Verification items for the finished model (mm, model axes). Round coordinates to 2 decimals unless told otherwise and drop trailing zeros. Write each loop counter-clockwise with the first axis right and the second up, starting at its lowest first coordinate (ties: lowest second). Pieces come first, ordered by that corner, then holes. Notation, with made-up numbers: (81.25, 51.25) -> (86.25, 51.25) arc R26 cw to (86.25, 77.25) -> close; hole circle Ø3 at (47.25, 50). An arc over 180 degrees is marked (long way). Answer as a JSON object with one key per item and string values. Group by question number.
(1) Sectioned sample at A-A on y = -5. Record the cut outline in (x, z) (3 decimals), and give its area (3 significant figures).
(2) Scan lines: L1, parallel to X at y = 35, z = -1 (3 decimals); L2, parallel to Y at x = 84.5, z = -0.8; L3, parallel to X at y = 34, z = -0.4. Record each from-to range of solid material in increasing order. Write a range as from..to.
(3) Sectioned sample at D-D on z = -1.35. Count the separate pieces of the cut face and the enclosed holes in it, and give its area (3 significant figures).
(4) Gauge pin test, flat ends, axial feed: pin 1 Ø5 at (x, y) = (-114.625, 55.25) entering from +Z; pin 2 Ø24 at (x, y) = (90.125, 74) entering from +Z. Record the tip position at first contact, or that the pin passes through.
(5) Sectioned sample at B-B on x = 12.5. Record the cut outline in (y, z) (3 decimals).
(6) Sectioned sample at C-C on y = 65. Record the cut outline in (x, z) (3 decimals).
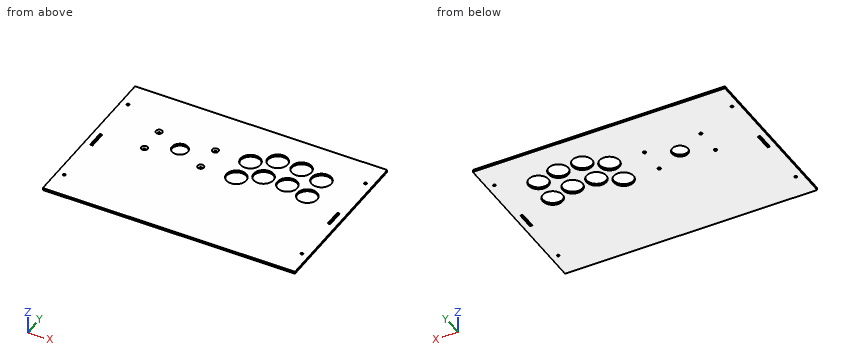
Autodesk Inventor part; units mm, degrees
ref_plane "YZ Plane" through (0, 0, 0) normal (1, 0, 0) x (0, 1, 0)
ref_plane "XZ Plane" through (0, 0, 0) normal (0, 1, 0) x (-1, 0, 0)
ref_plane "XY Plane" through (0, 0, 0) normal (0, 0, 1) x (1, 0, 0)
sketch "Panel" plane through (0, 0, 0) normal (0, 0, 1) x (1, 0, 0)
  line L0 (-190.5, 127) -> (190.5, 127)
  line L1 (190.5, 127) -> (190.5, -127)
  line L2 (190.5, -127) -> (-190.5, -127)
  line L3 (-190.5, -127) -> (-190.5, 127)
  point P0 (0, 0)
  point P1 (-190.5, 0)
  point P2 (0, 127)
  dimension "d0" = 254
  dimension "d3" = 381
sketch "JoystickMount" plane through (0, 0, 0) normal (0, 0, 1) x (1, 0, 0)
  line L0 (-114.625, 55.25) -> (-114.625, 14.75) construction
  line L1 (-114.625, 14.75) -> (-29.625, 14.75) construction
  point P0 (0, 0)
  point P1 (-72.125, 35)
  point P2 (-29.625, 55.25)
  point P3 (-114.625, 35)
  point P4 (-72.125, 14.75)
  dimension "d4" = 40.5
  dimension "d6" = 85
  dimension "d19" = 35
  dimension "d45" = 72.125
sketch "ButtonMounts" plane through (0, 0, 0) normal (0, 0, 1) x (1, 0, 0)
  line L0 (54.125, 74) -> (54.125, 35) construction
  line L1 (54.125, 35) -> (90.125, 35) construction
  point P0 (0, 0)
  point P1 (22.875, 56)
  point P2 (22.875, 17)
  point P3 (90.125, 74)
  point P4 (125.125, 65)
  point P5 (125.125, 26)
  point P6 (-72.125, 35)
  point P7 (72.125, 54.5)
  point P8 (54.125, 54.5)
  point P9 (72.125, 35)
  dimension "d7" = 39
  dimension "d9" = 39
  dimension "d10" = 39
  dimension "d11" = 39
  dimension "d12" = 31.25
  dimension "d13" = 36
  dimension "d14" = 35
  dimension "d15" = 18
  dimension "d16" = 9
  dimension "d55" = 144.25
  dimension "d56" = 72.125
extrude "PanelExtrusion" add sketch "Panel" against normal blind 3.175
hole "JoystickScrews" at (-29.625, 14.75, 0) at (-29.625, 55.25, 0) at (-114.625, 55.25, 0) at (-114.625, 14.75, 0) direction (0, 0, -1) diameter 4.5 end through all countersink diameter 9.4 countersink angle 90
hole "JoystickShaft" at (-72.125, 35, 0) direction (0, 0, -1) diameter 24 end through all
hole "ButtonHoles" at (125.125, 26, 0) at (90.125, 35, 0) at (90.125, 74, 0) at (125.125, 65, 0) at (54.125, 74, 0) at (54.125, 35, 0) at (22.875, 56, 0) at (22.875, 17, 0) direction (0, 0, -1) diameter 30 end through all
fillet "Corners" radius 1 4 edges at (190.5, 127, -1.5875) (190.5, -127, -1.5875) (-190.5, 127, -1.5875) (-190.5, -127, -1.5875)
ref_plane "10DegOffsetAlignment" through (190.5, -127, -3.175) normal (0, -0.9848, 0.1736) x (-1, 0, 0)
sketch "ScrewHoleCenters" plane through (0, 0, 0) normal (0, 0, 1) x (1, 0, 0)
  line L0 (-190.5, -126) -> (-190.5, 126)
  line L1 (-177.8, 89.411) -> (-180.975, 89.411)
  line L2 (-180.975, 85.6137) -> (-177.8, 85.6137)
  line L3 (-177.8, -85.9663) -> (-180.975, -85.9663)
  line L4 (-180.975, -89.7636) -> (-177.8, -89.7636)
  line L5 (177.8, -89.7636) -> (180.975, -89.7636)
  line L6 (180.975, -85.9663) -> (177.8, -85.9663)
  line L7 (177.8, 85.6137) -> (180.975, 85.6137)
  line L8 (180.975, 89.411) -> (177.8, 89.411)
  line L9 (-180.975, 89.411) -> (-180.975, 85.6137) construction
  line L10 (-177.8, 85.6137) -> (-177.8, 89.411) construction
  line L11 (-180.975, -85.9663) -> (-180.975, -89.7636) construction
  line L12 (-177.8, -89.7636) -> (-177.8, -85.9663) construction
  line L13 (177.8, -89.7636) -> (177.8, -85.9663) construction
  line L14 (180.975, -85.9663) -> (180.975, -89.7636) construction
  line L15 (177.8, 85.6137) -> (177.8, 89.411) construction
  line L16 (180.975, 89.411) -> (180.975, 85.6137) construction
  point P0 (0, 0)
  point P1 (-179.3875, 87.5123)
  point P2 (-177.8, 87.5123)
  point P3 (-179.3875, 85.6137)
  point P4 (-179.3875, -87.865)
  point P5 (179.3875, -87.865)
  point P6 (179.3875, 87.5123)
  point P7 (-179.3875, -89.7636)
  point P8 (-180.975, -87.865)
  point P9 (177.8, -87.865)
  point P10 (179.3875, -89.7636)
  point P11 (179.3875, 85.6137)
  point P12 (177.8, 87.5123)
hole "PanelBoltHoles" at (-179.3875, 87.5123, 0) at (-179.3875, -87.865, 0) at (179.3875, -87.865, 0) at (179.3875, 87.5123, 0) direction (0, 0, -1) diameter 3.7973 end through all
sketch "TabSlotSketch" plane through (0, 0, 0) normal (0, 0, 1) x (1, 0, 0)
  circle A0 centre (179.3875, -87.865) radius 1.8986
  circle A1 centre (-179.3875, 87.5123) radius 1.8986
  circle A2 centre (-179.3875, -87.865) radius 1.8986
  circle A3 centre (179.3875, 87.5123) radius 1.8986
  line L0 (190.5, 126) -> (190.5, -126)
  line L1 (-190.5, -126) -> (-190.5, 126)
  line L2 (-179.3875, 87.5123) -> (-179.3875, -87.865) construction
  line L3 (179.3875, 87.5123) -> (179.3875, -87.865) construction
  line L4 (-181.2798, 13.2095) -> (-177.4952, 13.2095)
  line L5 (-177.4952, 13.2095) -> (-177.4952, -13.5621)
  line L6 (-177.4952, -13.5621) -> (-181.2798, -13.5621)
  line L7 (-181.2798, -13.5621) -> (-181.2798, 13.2095)
  line L8 (181.2798, -13.5621) -> (177.4952, -13.5621)
  line L9 (177.4952, -13.5621) -> (177.4952, 13.2095)
  line L10 (177.4952, 13.2095) -> (181.2798, 13.2095)
  line L11 (181.2798, 13.2095) -> (181.2798, -13.5621)
  point P0 (0, 0)
  point P1 (-179.3875, -0.1763)
  point P2 (-181.2798, -0.1763)
  point P3 (-179.3875, -13.5621)
  point P4 (179.3875, -0.1763)
  point P5 (181.2798, -0.1763)
  point P6 (179.3875, 13.2095)
  point P7 (-179.3875, -0.1763)
  point P8 (179.3875, -0.1763)
  dimension "d66" = 26.7716
  dimension "d68" = 3.7846
  dimension "d69" = 26.7716
  dimension "d70" = 3.7846
extrude "TabSlotExtrusion" cut sketch "TabSlotSketch" against normal blind 3.175 contours L4 L5 L6 L7 | L8 L9 L10 L11
fillet "TabSlotFillets" radius 0.5 8 edges at (-177.4952, 13.2095, -1.5875) (-181.2798, 13.2095, -1.5875) (-177.4952, -13.5621, -1.5875) (-181.2798, -13.5621, -1.5875) (181.2798, 13.2095, -1.5875) (177.4952, 13.2095, -1.5875) (177.4952, -13.5621, -1.5875) (181.2798, -13.5621, -1.5875)
equation "\"d59\" = ScrewHoleD"
equation "\"d66\" = SlotLength"
equation "\"d68\" = SlotWidth"
equation "\"d69\" = SlotLength"
equation "\"d70\" = SlotWidth"
equation "\"d73\" = SlotFilletRad"
properties part number "Panel_top_2" material "Aluminum"
Computed values:
{
 "1": {"outline": "(-190.5, -3.175) -> (-181.28, -3.175) -> (-181.28, 0) -> (-190.5, 0) -> close; (-177.495, -3.175) -> (177.495, -3.175) -> (177.495, 0) -> (-177.495, 0) -> close; (181.28, -3.175) -> (190.5, -3.175) -> (190.5, 0) -> (181.28, 0) -> close", "area": "1,190 mm2"},
 "2": {"L1": "-190.5..-84.125, -60.125..39.125, 69.125..75.125, 105.125..113.125, 137.125..190.5", "L2": "-127..21.09, 48.91..60.09, 87.91..127", "L3": "-190.5..-84.08, -60.17..39.16, 69.09..75.16, 105.09..112.44, 137.81..190.5"},
 "3": {"separate pieces": "1", "enclosed holes": "19", "area": "90,300 mm2"},
 "4": {"pin 1": "z = -2.2", "pin 2": "through"},
 "5": {"outline": "(-127, -3.175) -> (6.167, -3.175) -> (6.167, 0) -> (-127, 0) -> close; (27.833, -3.175) -> (45.167, -3.175) -> (45.167, 0) -> (27.833, 0) -> close; (66.833, -3.175) -> (127, -3.175) -> (127, 0) -> (66.833, 0) -> close"},
 "6": {"outline": "(-190.5, -3.175) -> (10.875, -3.175) -> (10.875, 0) -> (-190.5, 0) -> close; (34.875, -3.175) -> (42.125, -3.175) -> (42.125, 0) -> (34.875, 0) -> close; (66.125, -3.175) -> (78.125, -3.175) -> (78.125, 0) -> (66.125, 0) -> close; (102.125, -3.175) -> (110.125, -3.175) -> (110.125, 0) -> (102.125, 0) -> close; (140.125, -3.175) -> (190.5, -3.175) -> (190.5, 0) -> (140.125, 0) -> close"}
}
